Input: part model. Units: mm. Frame: model coordinates. Face numbers are marked on the shaded views. A direction names the side the tool comes from. Round coordinates to 2 decimals unless told otherwise and drop trailing zeros. Order: outer loops, then holes, each group sorted by start corner. A loop starts at its lowest first (then second) coordinate and runs counter-clockwise, first axis right, second up. Notation, with made-up numbers: (19, 89) -> (66, 89) arc R13 ccw to (66, 103) -> close; hole circle Ø7 at (47.5, 72). An arc over 180 degrees is marked (long way). Use a Markdown table: item, result.
from build123d import *

# Parameters (mm, degrees)
SKETCH_1_R          = 7
EXTRUDE_1_DEPTH     = 55
CUT_EXTRUDE_START   = -43
SKETCH_2_R          = 7
SKETCH_2_R_2        = 5
CUT_EXTRUDE_2_DEPTH = 43


with BuildPart() as part:
    # 草图1 → 凸台-拉伸1 (new body)
    with BuildSketch(Plane(origin=(0, 0, 0), x_dir=(1, 0, 0), z_dir=(0, 1, 0))):
        with Locations(Location((0, 0, 0), (0, 0, 270))):
            Circle(SKETCH_1_R)
    extrude(amount=EXTRUDE_1_DEPTH)

    # 草图2 → 切除-拉伸2 (cut)
    with BuildSketch(Plane(origin=(0, 55, 0), x_dir=(1, 0, 0), z_dir=(0, 1, 0)).offset(CUT_EXTRUDE_START)):
        with Locations(Location((0, 0, 0), (0, 0, 270))):
            Circle(SKETCH_2_R)
        with Locations(Location((0, 0, 0), (0, 0, 270))):
            Circle(SKETCH_2_R_2, mode=Mode.SUBTRACT)
    extrude(amount=CUT_EXTRUDE_2_DEPTH, mode=Mode.SUBTRACT)

    # 草图8 → 切除-旋转25 (revolve, cut)
    with BuildSketch(Plane.XY, mode=Mode.PRIVATE) as cut_revolve_25_sk:
        Polygon((-7, 9.974534831), (-6.231936672, 9.974534831), (-0.307906931, 0), (-7, 0), align=None)
    revolve(cut_revolve_25_sk.sketch.rotate(Axis((0, 0, 0), (0, 1, 0)), 270), axis=Axis((0, 0, 0), (0, 1, 0)), mode=Mode.SUBTRACT)


solid = part.part
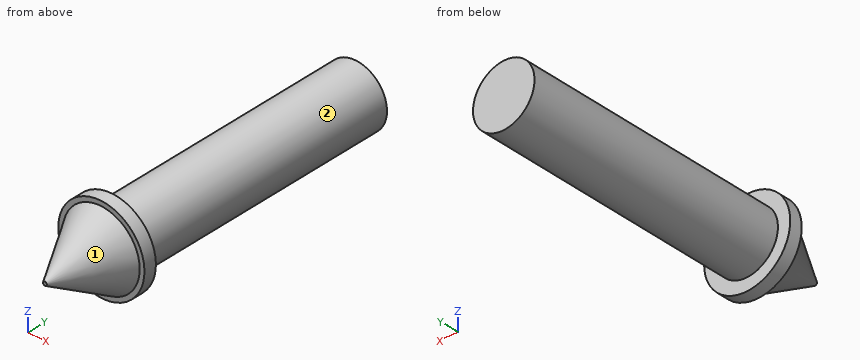
1) Cut plane A-A on y = 46.5. Return loops of the section in (x, z), and give its area (3 significant figures).
Results found:
| item | result |
|---|---|
| outline | circle Ø10 at (0, 0) |
| area | 78.5 mm² |
2) Cut plane B-B on y = 10.5. Return loops of the section in (x, z), and give its area (3 significant figures).
Results found:
| item | result |
|---|---|
| outline | circle Ø14 at (0, 0) |
| area | 154 mm² |
3) Set-up query: the marked faces 1 and 2. Return all of +Z, -Z, +X, -X, +Y, -Y with unobstructed straight access to the full face (end or side cutting, diameter ignored); none if empty.
Results found:
| item | result |
|---|---|
| face 1 | -Y |
| face 2 | +Y |
4) Line query: L1, parallel to X at y = 46, z = 0.25; L2, parallel to Y at x = -1.75, z = -6.5; L3, parallel to Z at x = 1.25, y = 25. Output: solid intervals per line, ascending. Write a range as [from, to].
Results found:
| item | result |
|---|---|
| L1 | x = [-4.99, 4.99] |
| L2 | y = [9.97, 12] |
| L3 | z = [-4.84, 4.84] |
5) Pin query (flat end, axial travel): pin 1 Ø2 at (x, y) = (4.5, 48.5) entering from -Z; pin 2 Ø1.5 at (x, z) = (3.5, -5) entering from +Y; pin 3 Ø6 at (x, y) = (-5, 34.5) entering from +Z. Return the tip coordinate at first contact, or that it passes through.
Results found:
| item | result |
|---|---|
| pin 1 | stops at z = -3.57 |
| pin 2 | stops at y = 12 |
| pin 3 | stops at z = 4.58 |
